Geometry check sheet. Reference: drawing and pictorial views, mm from the part's lowest x, y, z. A direction names the side the tool comes from. Give positions to 0.01 mm unless a question says otherwise; leave off trailing zeros. Write each loop counter-clockwise with the first axis right and the second up, starting at its lowest first coordinate (ties: lowest second). Pieces come first, ordered by that corner, then holes. Notation, with made-up numbers: M 8.5,-1.5 L 16.5,-1.5 A21 cw 16.5,19.5 Z; hole C 27.5,3.5 d7. An arc over 180 degrees is marked long. Answer as a JSON object with one key per item and string values.
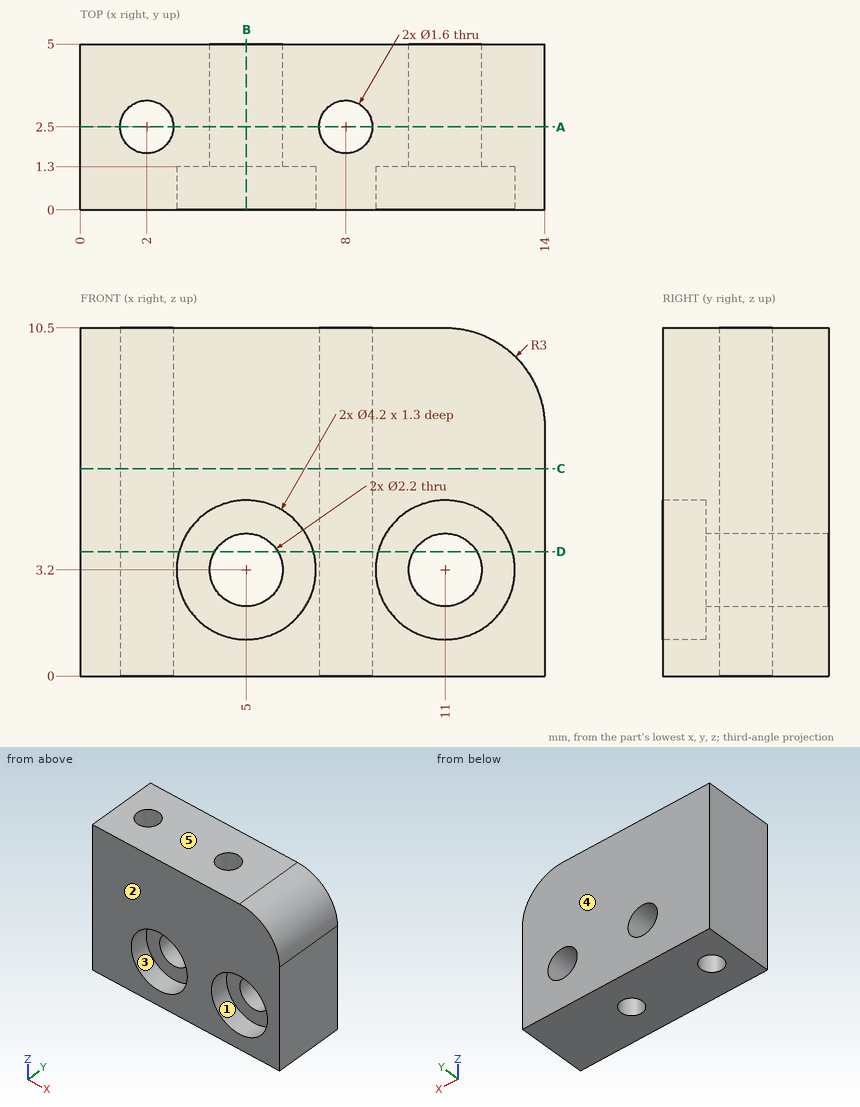
1) Section check B-B on x = 5. Record the boundary of the cut face in (y, z).
Completed:
{"outline": "M 0,0 L 5,0 L 5,2.1 L 1.3,2.1 L 1.3,1.1 L 0,1.1 Z; M 0,5.3 L 1.3,5.3 L 1.3,4.3 L 5,4.3 L 5,10.5 L 0,10.5 Z"}
2) Release check for a two-part mould opening along Z. For the marked faces 3, 4 and 5 record: pulls with the +Z half, pulls with the -Z half, needs draft (parallel to the pull), parting line crosses it, or undercut.
Completed:
{"face 3": "undercut", "face 4": "needs draft", "face 5": "pulls with the +Z half"}
3) Section check A-A on y = 2.5. Record the boundary of the cut face in (x, z).
Completed:
{"outline": "M 0,0 L 1.2,0 L 1.2,10.5 L 0,10.5 Z; M 2.8,0 L 7.2,0 L 7.2,10.5 L 2.8,10.5 Z; M 8.8,0 L 14,0 L 14,7.5 A3 ccw 11,10.5 L 8.8,10.5 Z; hole C 5,3.2 d2.2; hole C 11,3.2 d2.2"}
4) Section check C-C on z = 6.25. Record the boundary of the cut face in (x, y), and give its area (3 significant figures).
Completed:
{"outline": "M 0,0 L 14,0 L 14,5 L 0,5 Z; hole C 2,2.5 d1.6; hole C 8,2.5 d1.6", "area": "66.0 mm2"}
5) Thickness scan on L1, parallel to X at y = 2.15, z = 8.25; L2, parallel to Z at x = 11, y = 2.6; L3, parallel to X at y = 1.9, z = 5.75. Record the ranges inside material, lowest first.
Completed:
{"L1": "x = 0 to 1.28, 2.72 to 7.28, 8.72 to 13.9", "L2": "z = 0 to 2.1, 4.3 to 10.5", "L3": "x = 0 to 1.47, 2.53 to 7.47, 8.53 to 14"}
6) Section check D-D on z = 3.75. Record the boundary of the cut face in (x, y).
Completed:
{"outline": "M 0,0 L 2.97,0 L 2.97,1.3 L 4.05,1.3 L 4.05,5 L 0,5 Z; M 5.95,1.3 L 7.03,1.3 L 7.03,0 L 8.97,0 L 8.97,1.3 L 10.05,1.3 L 10.05,5 L 5.95,5 Z; M 11.95,1.3 L 13.03,1.3 L 13.03,0 L 14,0 L 14,5 L 11.95,5 Z; hole C 2,2.5 d1.6; hole C 8,2.5 d1.6"}
7) Go/stop test with flat-tipped pins: pin 1 (1.3 mm diameter, centred on x = 11, z = 2, fed in from -Y); pin 2 (1.8 mm diameter, centred on x = 2, y = 2.5, fed in from -Z); pin 3 (2 mm diameter, centred on x = 11, z = 3.2, fed in from +Y). Record where each tip stops, or that it passes through.
Completed:
{"pin 1": "stops at y = 1.3", "pin 2": "stops at z = 0", "pin 3": "passes through"}
8) Access from +Z, -Z, +X, -X, +Y, -Y to the whole of each face (thin tool, end or side, straight path). Record for the marked faces 1 and 2.
Completed:
{"face 1": "-Y", "face 2": "+Z, -Z, +X, -X, -Y"}
